Design review of the part built by this model. Coordinates are the model's own, in mm. A direction names the side the tool comes from. Give positions to 0.01 mm unless a question says otherwise; leave off trailing zeros. Order: outer loops, then holes, each group sorted by start corner. A loop starts at its lowest first (then second) coordinate and runs counter-clockwise, first axis right, second up. Notation, with made-up numbers: (-25, 76) -> (-15, 76) arc R26 cw to (-15, 114) -> close; hole circle Ø11 at (5, 40.5). An arc over 180 degrees is marked (long way). One line per item, written item: value. Start each with the question number.
1) Consider section B-B (z = -7.5). State the section outline as (x, y) points, plus the area to 3 significant figures.
2) Consider section A-A (z = -3.5). State how many separate pieces and enclosed holes the cut face has, plus the area to 3 significant figures.
3) Tool access review of faces 1 (the face through (-18.05, -20, -2)), 2 (the face through (-21, -22, 1)), 3 (the face through (-16, -18.718, -2)), 4 (the face through (-2.452, 1.52, 1.014)): name each direction out of +Z, -Z, +X, -X, +Y, -Y from which nothing blocks a thin tool from reaching the whole face with its end or side.
4) The part is to be moulded in two halves that separate along X. For faces 5 (the face through (-1.689, 9.856, 1.014)), 6 (the face through (0, 30, 1)), 7 (the face through (-14.97, -16, -2)), 8 (the face through (-16, -18, -5)), say which applies: released by +X, released by -X, zero draft, split by the parting line, or undercut.
5) Wall thickness on line 1 along Y through (x, z) = (-22.5, 1.45); line 2 along Y through (x, z) = (22.5, 0.55); line 3 along Z through (x, y) = (13, 20): over which ranges is each line inside the solid? List them lowest first. Write a range as from..to.
6) For pin 1 (0.9 mm diameter, centred on x = -17, z = -1.5, fed in from -Y); pin 2 (0.9 mm diameter, centred on x = -16.5, z = 1.5, fed in from -Y); pin 3 (2 mm diameter, centred on y = 7.5, z = -5.5, fed in from +X); pin 4 (3 mm diameter, centred on y = 9.5, z = -2.5, fed in from -X), all flat-tipped, find the tip position at first contact; note any pin that passes through.
7) Consider section C-C (y = -22.5). State the section outline as (x, z) points, plus the area to 3 significant figures.
from build123d import *

# Parameters (mm, degrees)
EXTRUDE_1_DEPTH     = 2
SKETCH_3_R          = 1.25
CUT_EXTRUDE_1_DEPTH = 2
SKETCH_4_R          = 2
CUT_EXTRUDE_2_DEPTH = 1
SKETCH_6_W          = 3.080004
SKETCH_6_H          = 6.793992
EXTRUDE_2_DEPTH     = 5
CUT_EXTRUDE_START   = -5
SKETCH_7_W          = 3.080004
SKETCH_7_H          = 0.5
CUT_EXTRUDE_4_DEPTH = 5
CUT_EXTRUDE_5_DEPTH = 5
SKETCH_9_W          = 3.080004
SKETCH_9_H          = 1.323498
CUT_EXTRUDE_6_DEPTH = 0.8
CUT_EXTRUDE_7_DEPTH = 3
SKETCH_11_W         = 1.5
SKETCH_11_H         = 0.5299964
SKETCH_11_H_2       = 0.5300218
CUT_EXTRUDE_8_DEPTH = 0.5
SKETCH_12_W         = 5.08
SKETCH_12_H         = 2.54
EXTRUDE_3_DEPTH     = 11


with BuildPart() as part:
    # 草图2 → 凸台-拉伸1 (new body)
    with BuildSketch(Plane.XY):
        with BuildLine():
            ThreePointArc((24.686269666, 24.686269666), (0, 30), (-24.686269666, 24.686269666))
            ThreePointArc((-24.686269666, 24.686269666), (-30, 0), (-24.686269666, -24.686269666))
            ThreePointArc((-24.686269666, -24.686269666), (0, -30), (24.686269666, -24.686269666))
            ThreePointArc((24.686269666, -24.686269666), (30, 0), (24.686269666, 24.686269666))
        make_face()
    extrude(amount=EXTRUDE_1_DEPTH)

    # 草图3 → 切除-拉伸1 (cut)
    with BuildSketch(Plane.XY.offset(2)):
        with Locations((-22.5, 22.5)):
            Circle(SKETCH_3_R)
        with Locations((22.5, 22.5)):
            Circle(SKETCH_3_R)
        with Locations((-22.5, -22.5)):
            Circle(SKETCH_3_R)
        with Locations((22.5, -22.5)):
            Circle(SKETCH_3_R)
    extrude(amount=-CUT_EXTRUDE_1_DEPTH, mode=Mode.SUBTRACT)

    # 草图4 → 切除-拉伸2 (cut)
    with BuildSketch(Plane.XY.offset(2)):
        with Locations((-22.5, 22.5)):
            Circle(SKETCH_4_R)
        with Locations((22.5, 22.5)):
            Circle(SKETCH_4_R)
        with Locations((22.5, -22.5)):
            Circle(SKETCH_4_R)
        with Locations((-22.5, -22.5)):
            Circle(SKETCH_4_R)
    extrude(amount=-CUT_EXTRUDE_2_DEPTH, mode=Mode.SUBTRACT)

    # 草图6 → 凸台-拉伸2 (add)
    with BuildSketch(Plane(origin=(0, 0, 0), x_dir=(-1, 0, 0), z_dir=(0, 0, -1))):
        with Locations((16.51, -17.145)):
            Rectangle(SKETCH_6_W, SKETCH_6_H)
    extrude(amount=EXTRUDE_2_DEPTH)

    # 草图7 → 切除-拉伸4 (cut)
    with BuildSketch(Plane(origin=(0, 0, -5), x_dir=(-1, 0, 0), z_dir=(0, 0, -1)).offset(CUT_EXTRUDE_START)):
        with Locations((16.51, -15.321502)):
            Rectangle(SKETCH_7_W, SKETCH_7_H)
        with Locations((16.51, -17.145)):
            Rectangle(SKETCH_7_W, SKETCH_7_H)
        with Locations((16.51, -18.968498)):
            Rectangle(SKETCH_7_W, SKETCH_7_H)
    extrude(amount=CUT_EXTRUDE_4_DEPTH, mode=Mode.SUBTRACT)

    # 草图8 → 切除-拉伸5 (cut)
    with BuildSketch(Plane.XY.offset(2)):
        with BuildLine():
            Line((4.91157439, 8.710708181), (-6.35957061, -7.717244434))
            ThreePointArc((-6.35957061, -7.717244434), (-5.720805987, -8.201974083), (-5.04525755, -8.633966427))
            Line((-5.04525755, -8.633966427), (6.239861639, 7.81435389))
            ThreePointArc((6.239861639, 7.81435389), (5.593701291, 8.289180048), (4.91157439, 8.710708181))
        make_face()
        with BuildLine():
            Line((-0.483946584, 9.988282921), (-9.493244962, -3.142976312))
            ThreePointArc((-9.493244962, -3.142976312), (-9.800391035, -1.988048178), (-9.967568149, -0.804726786))
            Line((-9.967568149, -0.804726786), (-2.836233135, 9.589357726))
            ThreePointArc((-2.836233135, 9.589357726), (-1.672029805, 9.859224936), (-0.483946584, 9.988282921))
        make_face()
        with BuildLine():
            Line((-5.705235003, 8.212812768), (-9.715721467, 2.367436669))
            ThreePointArc((-9.715721467, 2.367436669), (-8.245821975, 5.65742167), (-5.705235003, 8.212812768))
        make_face()
        with BuildLine():
            Line((9.578841572, 2.871549083), (0.767992477, -9.970465764))
            ThreePointArc((0.767992477, -9.970465764), (1.815657886, -9.833788001), (2.843055403, -9.587337272))
            Line((2.843055403, -9.587337272), (9.968138202, 0.797634494))
            ThreePointArc((9.968138202, 0.797634494), (9.828345995, 1.844888885), (9.578841572, 2.871549083))
        make_face()
        with BuildLine():
            Line((9.873157751, -1.587688896), (5.034385744, -8.64031019))
            ThreePointArc((5.034385744, -8.64031019), (8.245821975, -5.65742167), (9.873157751, -1.587688896))
        make_face()
        with BuildLine():
            Line((1.224216457, 9.924781815), (-8.819278945, -4.713843325))
            ThreePointArc((-8.819278945, -4.713843325), (-8.34274934, -5.513486506), (-7.793929004, -6.265354793))
            Line((-7.793929004, -6.265354793), (3.040773833, 9.52647335))
            ThreePointArc((3.040773833, 9.52647335), (2.141774487, 9.767947689), (1.224216457, 9.924781815))
        make_face()
        with BuildLine():
            Line((8.668880472, 4.985028723), (-1.53135707, -9.882051686))
            ThreePointArc((-1.53135707, -9.882051686), (-2.432490647, -9.699638614), (-3.313061985, -9.435232921))
            Line((-3.313061985, -9.435232921), (7.610812743, 6.4865653))
            ThreePointArc((7.610812743, 6.4865653), (8.174396358, 5.760142723), (8.668880472, 4.985028723))
        make_face()
    extrude(amount=-CUT_EXTRUDE_5_DEPTH, mode=Mode.SUBTRACT)

    # 草图9 → 切除-拉伸6 (cut)
    with BuildSketch(Plane.XY.offset(2)):
        with Locations((-16.51, -14.409753)):
            Rectangle(SKETCH_9_W, SKETCH_9_H)
        with Locations((-16.51, -16.233251)):
            Rectangle(SKETCH_9_W, SKETCH_9_H)
        with Locations((-16.51, -18.056749)):
            Rectangle(SKETCH_9_W, SKETCH_9_H)
        with Locations((-16.51, -19.880247)):
            Rectangle(SKETCH_9_W, SKETCH_9_H)
    extrude(amount=-CUT_EXTRUDE_6_DEPTH, mode=Mode.SUBTRACT)

    # 草图10 → 切除-拉伸7 (cut)
    with BuildSketch(Plane.XY.offset(2)):
        Polygon((-11.1005, -12.1700036), (-11.1005, -12.7), (-12.827, -12.7), (-12.827, -15.24), (-11.1005, -15.24), (-11.1005, -15.7700218), (-13.3369812, -15.7700218), (-13.3369812, -12.1700036), align=None)
        Polygon((-7.2369934, -12.1700036), (-7.2369934, -15.7700218), (-9.6005, -15.7700218), (-9.6005, -15.24), (-7.747, -15.24), (-7.747, -12.7), (-9.6005, -12.7), (-9.6005, -12.1700036), align=None)
        Polygon((12.5709934, 11.9600218), (14.9345, 11.9600218), (14.9345, 11.43), (13.081, 11.43), (13.081, 8.89), (14.9345, 8.89), (14.9345, 8.3600036), (12.5709934, 8.3600036), align=None)
        Polygon((18.6709812, 11.9600218), (18.6709812, 8.3600036), (16.4345, 8.3600036), (16.4345, 8.89), (18.161, 8.89), (18.161, 11.43), (16.4345, 11.43), (16.4345, 11.9600218), align=None)
    extrude(amount=-CUT_EXTRUDE_7_DEPTH, mode=Mode.SUBTRACT)

    # 草图11 → 切除-拉伸8 (cut)
    with BuildSketch(Plane.XY.offset(2)):
        with Locations((-10.3505, -12.4350018)):
            Rectangle(SKETCH_11_W, SKETCH_11_H)
        with Locations((-10.3505, -15.5050109)):
            Rectangle(SKETCH_11_W, SKETCH_11_H_2)
        with Locations((15.6845, 11.6950109)):
            Rectangle(SKETCH_11_W, SKETCH_11_H_2)
        with Locations((15.6845, 8.6250018)):
            Rectangle(SKETCH_11_W, SKETCH_11_H)
    extrude(amount=-CUT_EXTRUDE_8_DEPTH, mode=Mode.SUBTRACT)

    # 草图12 → 凸台-拉伸3 (add)
    with BuildSketch(Plane(origin=(0, 0, 0), x_dir=(-1, 0, 0), z_dir=(0, 0, -1))):
        with Locations((-15.621, 10.16)):
            Rectangle(SKETCH_12_W, SKETCH_12_H)
        with Locations((10.287, -13.97)):
            Rectangle(SKETCH_12_W, SKETCH_12_H)
    extrude(amount=EXTRUDE_3_DEPTH)


solid = part.part
Checked values:
1. outline: (-12.83, -15.24) -> (-7.75, -15.24) -> (-7.75, -12.7) -> (-12.83, -12.7) -> close; (13.08, 8.89) -> (18.16, 8.89) -> (18.16, 11.43) -> (13.08, 11.43) -> close
1. area: 25.8 mm^2
2. separate pieces: 6
2. enclosed holes: 0
2. area: 42.1 mm^2
3. face 1: -Z, -X, +Y, -Y
3. face 2: +Z
3. face 3: -Z, +X, -X
3. face 4: +Z, -Z
4. face 5: undercut
4. face 6: split by the parting line
4. face 7: released by +X
4. face 8: zero draft
5. line 1: y = -25.62..-24.5, -20.5..20.5, 24.5..25.62
5. line 2: y = -25.62..-23.75, -21.25..21.25, 23.75..25.62
5. line 3: z = 0..2
6. pin 1: stops at y = -20.54
6. pin 2: stops at y = -27.81
6. pin 3: passes through
6. pin 4: stops at x = 13.08
7. outline: (-25.62, 0) -> (-23.75, 0) -> (-23.75, 1) -> (-24.5, 1) -> (-24.5, 2) -> (-25.62, 2) -> close; (-21.25, 0) -> (21.25, 0) -> (21.25, 1) -> (20.5, 1) -> (20.5, 2) -> (-20.5, 2) -> (-20.5, 1) -> (-21.25, 1) -> close; (23.75, 0) -> (25.62, 0) -> (25.62, 2) -> (24.5, 2) -> (24.5, 1) -> (23.75, 1) -> close
7. area: 89.5 mm^2
